```python
from build123d import *

# Parameters (mm, degrees)
ESQUISSE1_W             = 45
ESQUISSE1_H             = 22
BOSS_EXTRU_1_DEPTH      = 5
ESQUISSE2_R             = 1.2
ENL_V_MAT_EXTRU_1_DEPTH = 32.862987933


with BuildPart() as part:
    # Esquisse1 → Boss.-Extru.1 (new, symmetric)
    with BuildSketch(Plane(origin=(0, 0, 0), x_dir=(1, 0, 0), z_dir=(0, 1, 0))):
        with Locations((0, -11)):
            Rectangle(ESQUISSE1_W, ESQUISSE1_H)
    extrude(amount=BOSS_EXTRU_1_DEPTH, both=True)

    # Esquisse2 → Enlèv. mat.-Extru.1 (cut, through all)
    with BuildSketch(Plane.XY.offset(22)):
        with Locations((-15, 0)):
            Circle(ESQUISSE2_R)
        with Locations((15, 0)):
            Circle(ESQUISSE2_R)
    extrude(amount=-ENL_V_MAT_EXTRU_1_DEPTH, mode=Mode.SUBTRACT)


solid = part.part
```
Part model, mm, in its own coordinate system. Round coordinates to 2 decimals unless told otherwise and drop trailing zeros. Order: outer loops, then holes, each group sorted by start corner. A loop starts at its lowest first (then second) coordinate and runs counter-clockwise, first axis right, second up. Notation, with made-up numbers: M 0,-1.5 L 34,-1.5 A31 cw 34,29.5 Z; hole C -6,33 d1. An arc over 180 degrees is marked long. Put each result on its own line as item: value. Start each with the question number.
1. Drill centre lines: probe 1 along Y at (x, z) = (15, 9.25); probe 2 along X at (y, z) = (-0.5, 21); probe 3 along X at (y, z) = (-1, 5). Where is each one in solid material? Low to high. Write a range as [from, to].
2. Two-plate mould, pull along X, no slides. Class faces 1 (the face through (-22.5, 0, 11)), 2 (the face through (22.5, 0, 11)), 3 (the face through (-13.855, 0.36, 11.154)), 4 (the face through (0, 0, 22)): +X half, -X half, draft (parallel to the pull), parting line (faces both ways), or undercut.
3. Slice it at A-A on x = 15. List the corners of the cut face in (y, z), then the cut area to 3 significant figures.
4. Drop a flat-ended pin along its axis: pin 1 (1.4 mm diameter, centred on x = 15, y = 0, fed in from -Z). Give the stop position or say it passes through.
5. Slice it at B-B on y = 0. List the corners of the cut face in (x, z).
Findings:
1. probe 1: [-5, -1.2], [1.2, 5]
1. probe 2: [-22.5, -16.09], [-13.91, 13.91], [16.09, 22.5]
1. probe 3: [-22.5, -15.66], [-14.34, 14.34], [15.66, 22.5]
2. face 1: -X half
2. face 2: +X half
2. face 3: undercut
2. face 4: draft
3. outline: M -5,0 L -1.2,0 L -1.2,22 L -5,22 Z; M 1.2,0 L 5,0 L 5,22 L 1.2,22 Z
3. area: 167 mm2
4. pin 1: through
5. outline: M -22.5,0 L -16.2,0 L -16.2,22 L -22.5,22 Z; M -13.8,0 L 13.8,0 L 13.8,22 L -13.8,22 Z; M 16.2,0 L 22.5,0 L 22.5,22 L 16.2,22 Z
